```python
from build123d import *

# Parameters (mm, degrees)
SKETCH1_R           = 3.95
BOSS_EXTRUDE1_DEPTH = 3
FILLET1_R           = 0.5


with BuildPart() as part:
    # Sketch1 → Boss-Extrude1 (new body)
    with BuildSketch(Plane(origin=(0, 0, 0), x_dir=(1, 0, 0), z_dir=(0, 1, 0))):
        Circle(SKETCH1_R)
        with BuildLine():
            Line((-1.985572965, -1.6), (1.985572965, -1.6))
            ThreePointArc((1.985572965, -1.6), (0, 2.55), (-1.985572965, -1.6))
        make_face(mode=Mode.SUBTRACT)
    extrude(amount=BOSS_EXTRUDE1_DEPTH)

    # Fillet1
    fillet1_edges = [part.edges().sort_by_distance(p)[0] for p in [
        (-3.95, 0, 0),
        (-3.95, 3, 0),
        (0, 0, 1.6),
        (0, 3, 1.6),
    ]]
    fillet(fillet1_edges, radius=FILLET1_R)


solid = part.part
```
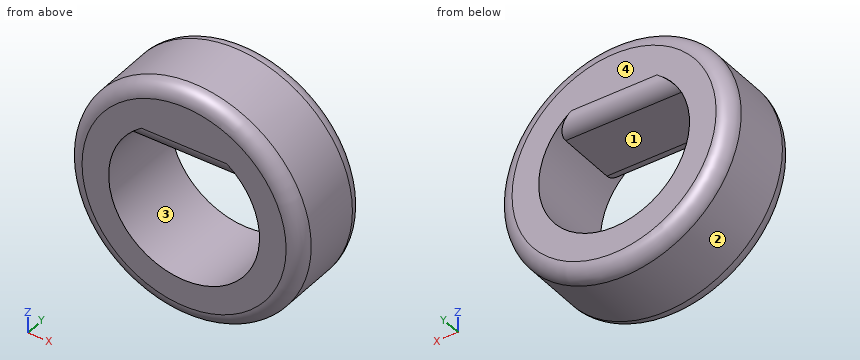
Geometry check sheet. Reference: the model listing, model coordinates, mm. Face numbers are marked on the shaded views. Give positions to 0.01 mm unless a question says otherwise; leave off trailing zeros. Order: outer loops, then holes, each group sorted by start corner. A loop starts at its lowest first (then second) coordinate and runs counter-clockwise, first axis right, second up.
1. Release check for a two-part mould opening along X. For the marked faces 1, 2, 3 and 4 record: pulls with the +X half, pulls with the -X half, needs draft (parallel to the pull), parting line crosses it, or undercut.
2. Section check C-C, the plane y = 1.3. Enter the section's corners in (x, z), and give its area (3 significant figures).
3. Thickness scan on L1, parallel to X at y = 1, z = 0; L2, parallel to Z at x = 0, y = 2.35; L3, parallel to X at y = 2.8, z = 1.5. Record the ranges inside material, lowest first.
4. Section check B-B, the plane z = 0. Enter the section's corners in (x, y), and give its area (3 significant figures).
5. Section check A-A, the plane x = 0. Enter the section's corners in (y, z), and give its area (3 significant figures).
6. Gauge pin test, flat end, axial feed: pin 1 Ø0.6 at (x, y) = (-0.5, 1) entering from -Z. Record the tip position at first contact, or that the pin passes through.
7. Section check D-D, the plane y = 2.75. Enter the section's corners in (x, z).
Values follow:
1. face 1: undercut
1. face 2: parting line crosses it
1. face 3: undercut
1. face 4: needs draft
2. outline: circle Ø7.9 at (0, 0); hole (-1.99, 1.6) arc R2.55 ccw (long way) to (1.99, 1.6) - close
2. area: 31.2 mm2
3. L1: x = -3.95 to -2.55, 2.55 to 3.95
3. L2: z = -3.95 to -2.55, 1.6 to 3.95
3. L3: x = -3.55 to -2.06, 2.06 to 3.55
4. outline: (-3.95, 0.5) arc R0.5 ccw to (-3.45, 0) - (-2.55, 0) - (-2.55, 3) - (-3.45, 3) arc R0.5 ccw to (-3.95, 2.5) - close; (2.55, 0) - (3.45, 0) arc R0.5 ccw to (3.95, 0.5) - (3.95, 2.5) arc R0.5 ccw to (3.45, 3) - (2.55, 3) - close
4. area: 8.19 mm2
5. outline: (0, -3.45) arc R0.5 ccw to (0.5, -3.95) - (2.5, -3.95) arc R0.5 ccw to (3, -3.45) - (3, -2.55) - (0, -2.55) - close; (0, 2.1) arc R0.5 ccw to (0.5, 1.6) - (2.5, 1.6) arc R0.5 ccw to (3, 2.1) - (3, 3.45) arc R0.5 ccw to (2.5, 3.95) - (0.5, 3.95) arc R0.5 ccw to (0, 3.45) - close
5. area: 10.9 mm2
6. pin 1: stops at z = -3.94
7. outline: circle Ø7.77 at (0, 0); hole (-1.93, 1.67) arc R2.55 ccw (long way) to (1.93, 1.67) - close
